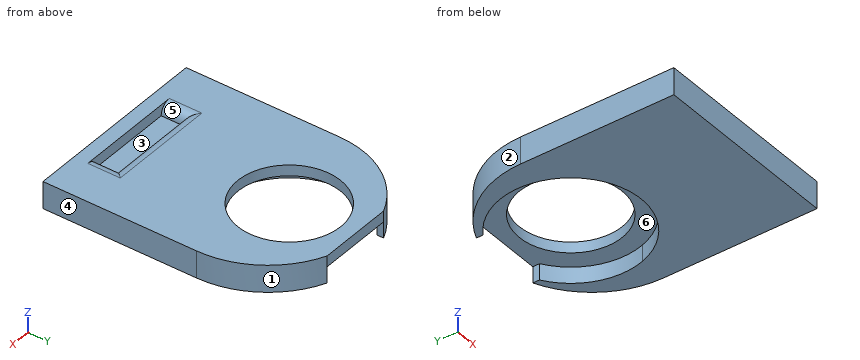
from build123d import *

# Parameters (mm, degrees)
BOSS_EXTRUDE1_DEPTH = 1.5
BOSS_EXTRUDE2_DEPTH = 1
SKETCH4_R           = 4.75
CUT_EXTRUDE1_DEPTH  = 23.898325822
SKETCH5_W           = 17.56
SKETCH5_H           = 2.5
BOSS_EXTRUDE3_DEPTH = 0.15
SKETCH6_W           = 17.56
SKETCH6_H           = 2.5
BOSS_EXTRUDE4_DEPTH = 7.5
SKETCH9_W           = 8
SKETCH9_H           = 2
CUT_EXTRUDE2_DEPTH  = 1
FILLET1_R           = 1


with BuildPart() as part:
    # Sketch1 → Boss-Extrude1 (new body)
    with BuildSketch(Plane.XY):
        with BuildLine():
            ThreePointArc((14.980604809, 6.55), (8.78, 2), (2.579395191, 6.55))
            Line((2.579395191, 6.55), (0, 6.55))
            Line((0, 6.55), (0, 0))
            Line((0, 0), (17.56, 0))
            Line((17.56, 0), (17.56, 6.55))
            Line((17.56, 6.55), (14.980604809, 6.55))
        make_face()
        with BuildLine():
            ThreePointArc((2.579395191, 6.55), (2.679421093, 10.743420825), (5.32, 14.002581212))
            Line((5.32, 14.002581212), (5.32, 14.619498126))
            ThreePointArc((5.32, 14.619498126), (1.449679407, 11.382680416), (0, 6.55))
            Line((0, 6.55), (2.579395191, 6.55))
        make_face()
        with BuildLine():
            ThreePointArc((12.24, 14.002581212), (14.880578907, 10.743420825), (14.980604809, 6.55))
            Line((14.980604809, 6.55), (17.56, 6.55))
            ThreePointArc((17.56, 6.55), (16.110320593, 11.382680416), (12.24, 14.619498126))
            Line((12.24, 14.619498126), (12.24, 14.002581212))
        make_face()
    extrude(amount=BOSS_EXTRUDE1_DEPTH)

    # Sketch3 → Boss-Extrude2 (add)
    with BuildSketch(Plane.XY.offset(1.5)):
        with BuildLine():
            Line((12.24, 14.619498126), (12.24, 14.002581212))
            ThreePointArc((12.24, 14.002581212), (8.78, 2), (5.32, 14.002581212))
            Line((5.32, 14.002581212), (5.32, 14.619498126))
            ThreePointArc((5.32, 14.619498126), (1.449679407, 11.382680416), (0, 6.55))
            Line((0, 6.55), (0, 0))
            Line((0, 0), (17.56, 0))
            Line((17.56, 0), (17.56, 6.55))
            ThreePointArc((17.56, 6.55), (16.110320593, 11.382680416), (12.24, 14.619498126))
        make_face()
        with BuildLine():
            Line((5.32, 14.619498126), (12.24, 14.619498126))
            Line((12.24, 14.619498126), (12.24, 14.002581212))
            ThreePointArc((12.24, 14.002581212), (8.78, 2), (5.32, 14.002581212))
            Line((5.32, 14.002581212), (5.32, 14.619498126))
        make_face()
    extrude(amount=BOSS_EXTRUDE2_DEPTH)

    # Sketch4 → Cut-Extrude1 (cut, through all)
    with BuildSketch(Plane(origin=(0, 0, 1.5), x_dir=(-1, 0, 0), z_dir=(0, 0, -1))):
        with Locations((-8.78, 8.5)):
            Circle(SKETCH4_R)
    extrude(amount=-CUT_EXTRUDE1_DEPTH, mode=Mode.SUBTRACT)

    # Sketch5 → Boss-Extrude3 (add)
    with BuildSketch(Plane.XZ):
        with Locations((8.78, 1.25)):
            Rectangle(SKETCH5_W, SKETCH5_H)
    extrude(amount=BOSS_EXTRUDE3_DEPTH)

    # Sketch6 → Boss-Extrude4 (add)
    with BuildSketch(Plane.XZ.offset(0.15)):
        with Locations((8.78, 1.25)):
            Rectangle(SKETCH6_W, SKETCH6_H)
    extrude(amount=BOSS_EXTRUDE4_DEPTH)

    # Sketch9 → Cut-Extrude2 (cut)
    with BuildSketch(Plane.XY.offset(2.5)):
        with Locations((8.78, -5.353166831)):
            Rectangle(SKETCH9_W, SKETCH9_H)
    extrude(amount=-CUT_EXTRUDE2_DEPTH, mode=Mode.SUBTRACT)

    # Fillet1
    fillet1_edges = [part.edges().sort_by_distance(p)[0] for p in [
        (4.78, -5.353166831, 2.5),
        (12.78, -5.353166831, 2.5),
        (8.78, -4.353166831, 2.5),
    ]]
    fillet(fillet1_edges, radius=FILLET1_R - 0.0001)  # a hair under: the kernel refuses the full size


solid = part.part
Geometry: final body of the model. Coordinates: model frame, mm. Face numbers are marked on the shaded views. A direction names the side the tool comes from. Round coordinates to 2 decimals unless told otherwise and drop trailing zeros. Loops run counter-clockwise (first coordinate to the right, second up) from the corner with the lowest first, then second, coordinate; pieces in that order, holes last. Notation, with made-up numbers: M 69.5,57 L 73.5,57 A15 ccw 73.5,81 Z; hole C -25.5,58 d11. An arc over 180 degrees is marked long. Put each result on its own line as item: value. Start each with the question number.
(1) Material intervals for line 1 along Y through (x, z) = (8.78, 2.3); line 2 along Z through (x, y) = (11.25, 13); line 3 along Y through (x, z) = (8.78, 1.9), sorted ascending. Write a range as [from, to].
(2) Section query C-C (z = 0.75). Return loops of the section in (x, y).
(3) Set-up query: the marked faces 4, 5 and 6. Return all of +Z, -Z, +X, -X, +Y, -Y with unobstructed straight access to the full face (end or side cutting, diameter ignored); none if empty.
(4) Draft query along X for the marked faces 1, 2 and 3. Return one class per face: +X half, -X half, draft (parallel to the pull), parting line (faces both ways), or undercut.
(5) Section query B-B (y = 9.75). Return loops of the section in (x, z).
(6) Section query D-D (x = 14.75). Return loops of the section in (y, z).
(7) Contact query for flat-ended pins moving along their axis: pin 1 Ø1.5 at (y, z) = (12, 1.5) entering from -X; pin 2 Ø0.7 at (y, z) = (14.5, 0.5) entering from +X; pin 3 Ø1 at (x, y) = (8.5, -5.5) entering from +Z. Output: stop coordinate, or through.
Findings below:
1. line 1: y = [-7.65, -6.35], [-3.95, 3.75], [13.25, 14.62]
1. line 2: z = [1.5, 2.5]
1. line 3: y = [-7.65, -6.35], [-4.27, 3.75], [13.25, 14.62]
2. outline: M 0,-7.65 L 17.56,-7.65 L 17.56,6.55 A8.78 ccw 12.24,14.62 L 12.24,14 A6.5 cw long 5.32,14 L 5.32,14.62 A8.78 ccw 0,6.55 Z
3. face 4: +Z, -Z, +X, +Y, -Y
3. face 5: +Z
3. face 6: -Z
4. face 1: +X half
4. face 2: -X half
4. face 3: undercut
5. outline: M 0.6,0 L 2.4,0 L 2.4,1.5 L 4.2,1.5 L 4.2,2.5 L 0.6,2.5 Z; M 13.36,1.5 L 15.16,1.5 L 15.16,0 L 16.96,0 L 16.96,2.5 L 13.36,2.5 Z
6. outline: M -7.65,0 L 5.93,0 L 5.93,1.5 L 11.07,1.5 L 11.07,0 L 12.99,0 L 12.99,2.5 L -7.65,2.5 Z
7. pin 1: stops at x = 1.36
7. pin 2: stops at x = 13.18
7. pin 3: stops at z = 1.5
